Work out the finished part from the listing and answer in its coordinate system (mm). A direction names the side the tool comes from. Round coordinates to 2 decimals unless told otherwise and drop trailing zeros. Write each loop counter-clockwise with the first axis right and the second up, starting at its lowest first coordinate (ties: lowest second). Pieces come first, ordered by that corner, then holes. Notation, with made-up numbers: M 29,80 L 60,80 A33 cw 60,110 Z; hole C 56.5,-8.75 d2. An arc over 180 degrees is marked long. Answer in a Markdown table with one row per item.
```python
from build123d import *

# Parameters (mm, degrees)
F1_DEPTH = 105
F2_R     = 12
F2_R_2   = 7
F3_DEPTH = 0.01
F4_W     = 50
F4_H     = 30
F5_DEPTH = 0.01
F6_DEPTH = 20


# Not quite as in the source:
# - ends of sketch curves that miss each other by under 0.0002 mm in the source are joined


with BuildPart() as f1:
    # F0 (on Front) → F1 (new body, symmetric)
    with BuildSketch(Plane.XZ):
        with BuildLine():
            Line((4.4999999997, -23.5), (4.4999999997, -30.5))
            ThreePointArc((4.4999999997, -30.5), (5.9644660938, -34.0355339059), (9.4999999997, -35.5))
            Line((9.4999999997, -35.5), (12.5, -35.5))
            ThreePointArc((12.5, -35.5), (13.9142133287, -34.9142135624), (14.4999997663, -33.5))
            Line((14.4999997663, -33.5), (14.4999997663, 22.4999994828))
            ThreePointArc((14.4999997663, 22.4999994828), (12.4539129776, 29.7872458033), (6.9137199183, 34.9444437777))
            ThreePointArc((6.9137199183, 34.9444437777), (5.8016169865, 35.3591259101), (4.6231056877, 35.4999993303))
            Line((4.6231056877, 35.4999993303), (3.4999997663, 35.4999993303))
            ThreePointArc((3.4999997663, 35.4999993303), (2.0857862039, 34.9142128927), (1.4999997663, 33.4999993303))
            Line((1.4999997663, 33.4999993303), (1.4999997663, 30.2459664828))
            ThreePointArc((1.4999997663, 30.2459664828), (1.7397477835, 29.4324771221), (2.3823530195, 28.8790310431))
            ThreePointArc((2.3823530195, 28.8790310431), (-0.5000000985, 15.4999997293), (-3.3823532363, 28.8790310342))
            ThreePointArc((-3.3823532363, 28.8790310342), (-2.7397478169, 29.4324771961), (-2.4999997997, 30.2459665567))
            Line((-2.4999997997, 30.2459665567), (-2.4999997997, 33.5))
            ThreePointArc((-2.4999997997, 33.5), (-3.0857862373, 34.9142132361), (-4.4999997997, 35.4999996738))
            Line((-4.4999997997, 35.4999996738), (-4.6231058319, 35.4999996738))
            ThreePointArc((-4.6231058319, 35.4999996738), (-5.8016171306, 35.3591262536), (-6.9137200625, 34.9444441212))
            ThreePointArc((-6.9137200625, 34.9444441212), (-14.4718653147, 21.6128794539), (-5.288282, 9.344303))
            Line((-5.288282, 9.344303), (1.210101, 6.979085))
            ThreePointArc((1.210101, 6.979085), (3.5957603078, 5.1485040574), (4.4999999997, 2.2806219993))
            Line((4.4999999997, 2.2806219993), (4.4999999997, 0.5))
            Line((4.4999999997, 0.5), (4.4999999997, -23.5))
        make_face()
    extrude(amount=F1_DEPTH, both=True)

    # F2 (on face) → F3 (join)
    with BuildSketch(Plane(origin=(4.4999999997, 0, 0), x_dir=(0, -1, 0), z_dir=(-1, 0, 0))):
        with Locations((0, -11.5)):
            Circle(F2_R)
        with Locations((0, -11.5)):
            Circle(F2_R_2, mode=Mode.SUBTRACT)
    extrude(amount=F3_DEPTH)

    # F4 (on face) → F5 (join)
    with BuildSketch(Plane.YZ.offset(14.4999997663)):
        with Locations((0, -17.5000005172)):
            Rectangle(F4_W, F4_H)
    extrude(amount=F5_DEPTH)

    # F6 (cut): a face of the model
    f6_faces = [f1.faces().sort_by_distance(p)[0] for p in [
        (4.4999999997, 0, -11.5),
    ]]
    extrude(f6_faces, amount=-F6_DEPTH, mode=Mode.SUBTRACT)


solid = f1.part
```
1. Consider line 1 along X through (y, z) = (-59.5, 30.5); line 2 along X through (y, z) = (-60.5, -7); line 3 along Z through (x, y) = (7.5, 0). Determine where each line is inside the solid, lowest interval first. Write a range as from..to.
Calculated:
| item | result |
|---|---|
| line 1 | x = -11.99..-2.5, 1.5..11.99 |
| line 2 | x = 4.5..14.5 |
| line 3 | z = -35.08..-18.5, -4.5..34.62 |
2. The part is cut by section D-D (y = 60.5). Determine the outline of the cut face in (x, z).
Calculated:
| item | result |
|---|---|
| outline | M -6.91,34.94 A14 ccw -5.29,9.34 L 1.21,6.98 A5 cw 4.5,2.28 L 4.5,-30.5 A5 ccw 9.5,-35.5 L 12.5,-35.5 A2 ccw 14.5,-33.5 L 14.5,22.5 A14 ccw 6.91,34.94 A5 ccw 4.62,35.5 L 3.5,35.5 A2 ccw 1.5,33.5 L 1.5,30.25 A1.5 ccw 2.38,28.88 A7 cw long -3.38,28.88 A1.5 ccw -2.5,30.25 L -2.5,33.5 A2 ccw -4.5,35.5 L -4.62,35.5 A5 ccw Z |
3. Determine the mould class of faces 1 (the cylindrical face through (-0.234, -1.47, 15.505)), 2 (the cylindrical face through (5.93, -1.47, -34)), 3 (the cylindrical face through (12.509, -1.47, 29.695)), 4 (the flat face through (4.5, -1, -25)) for opening direction Z: released by +Z, released by -Z, zero draft, split by the parting line, or undercut.
Calculated:
| item | result |
|---|---|
| face 1 | undercut |
| face 2 | released by -Z |
| face 3 | released by +Z |
| face 4 | zero draft |
4. Given pin 1 (6 mm diameter, centred on x = 9.5, y = 72.5, fed in from +Z); pin 2 (17 mm diameter, centred on y = -49.5, z = -1.5, fed in from +X); pin 3 (16 mm diameter, centred on y = 0, z = -11.5, fed in from -X); pin 4 (8.5 mm diameter, centred on y = 0, z = -11.5, fed in from -X), each flat-ended and moving along its own axis, determine where each tip first touches the part or whether it passes through.
Calculated:
| item | result |
|---|---|
| pin 1 | stops at z = 35.13 |
| pin 2 | stops at x = 14.5 |
| pin 3 | stops at x = 4.49 |
| pin 4 | passes through |
5. A tool of negligible diameter and unlimited length cuts with its end or side. For faces 5 (the flat face through (14.51, 0, -21)), 6 (the flat face through (4.49, -5, -17)), from which of +Z, -Z, +X, -X, +Y, -Y can it reach the whole face along a straight path? Write none if from no direction.
Calculated:
| item | result |
|---|---|
| face 5 | +Z, -Z, +X, +Y, -Y |
| face 6 | -Z, -X, +Y, -Y |
